from build123d import *

# Parameters (mm, degrees)
SKETCH1_R                = 2.159
BOSS_EXTRUDE2_DEPTH      = 2.54
BOSS_EXTRUDE5_DEPTH      = 25.4
BOSS_EXTRUDE5_DEPTH_BACK = 2.54
BOSS_EXTRUDE8_DEPTH      = 12.7
BOSS_EXTRUDE8_DEPTH_BACK = 2.54
SKETCH4_W                = 5.08
SKETCH4_H                = 2.54
BOSS_EXTRUDE9_DEPTH      = 5.08


with BuildPart() as part:
    # Sketch1 → Boss-Extrude2 (new body)
    with BuildSketch(Plane(origin=(0, 0, 0), x_dir=(1, 0, 0), z_dir=(0, 1, 0))):
        Polygon((0, -5.08), (5.08, -5.08), (10.489221848, 5.08), (43.764184298, 5.08), (51.562, -5.08), (61.722, -5.08), (61.722, 5.08), (56.642, 5.08), (51.562, 5.08), (46.152778152, 10.489221848), (10.489221848, 10.489221848), (5.08, 5.08), (-5.08, 5.08), (-5.08, -5.08), align=None)
        with Locations(Location((0, 0, 0), (0, 0, 270))):
            Circle(SKETCH1_R, mode=Mode.SUBTRACT)
        with Locations(Location((56.642, 0, 0), (0, 0, 270))):
            Circle(SKETCH1_R, mode=Mode.SUBTRACT)
    extrude(amount=BOSS_EXTRUDE2_DEPTH)

    # Sketch3 → Boss-Extrude5 (add, two sides: drawn at the far end of the back side and taken through both)
    with BuildSketch(Plane(origin=(0, 2.54, 0), x_dir=(1, 0, 0), z_dir=(0, 1, 0)).offset(-BOSS_EXTRUDE5_DEPTH_BACK)):
        Polygon((5.08, 12.7), (5.08, 5.08), (-5.08, 5.08), (-5.08, 12.7), (0, 12.7), align=None)
    extrude(amount=BOSS_EXTRUDE5_DEPTH + BOSS_EXTRUDE5_DEPTH_BACK)

    # Sketch4 → Boss-Extrude8 (add, two sides: drawn at the far end of the back side and taken through both)
    with BuildSketch(Plane(origin=(0, 2.54, 0), x_dir=(1, 0, 0), z_dir=(0, 1, 0)).offset(-BOSS_EXTRUDE8_DEPTH_BACK)):
        with Locations((29.878652905, 11.759221848)):
            Rectangle(SKETCH4_W, SKETCH4_H)
    extrude(amount=BOSS_EXTRUDE8_DEPTH + BOSS_EXTRUDE8_DEPTH_BACK)

    # Sketch7 → Boss-Extrude9 (add)
    with BuildSketch(Plane(origin=(32.418652905, 0, 0), x_dir=(0, 0, -1), z_dir=(1, 0, 0))):
        Polygon((10.489221848, 15.24), (5.391589044, 15.24), (5.391589044, 12.7), (5.391589044, 11.903510412), (7.271896049, 11.903510412), (8.703373283, 11.903510412), (8.703373283, 13.570272135), (7.703807283, 13.570272135), (7.703807283, 12.7), (7.271896049, 12.7), (6.661589044, 12.7), (5.865099456, 13.97), (6.661589044, 13.97), (10.489221848, 13.97), align=None)
    extrude(amount=-BOSS_EXTRUDE9_DEPTH)


solid = part.part
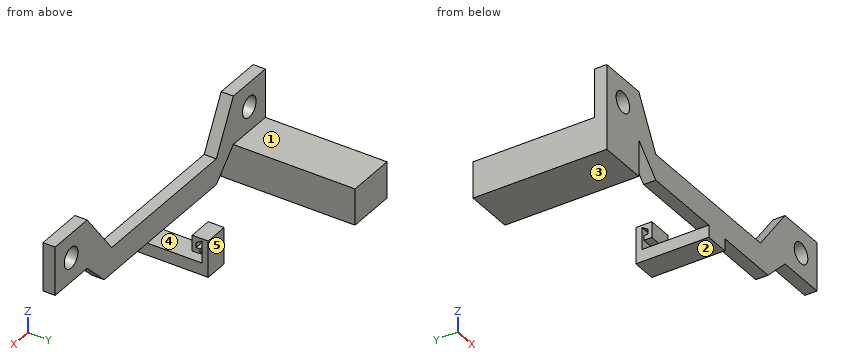
The model under review builds one solid part; all positions refer to its coordinate system, in mm. Face numbers are marked on the shaded views. A direction names the side the tool comes from. Coordinates: 2 decimals unless noted, no trailing zeros. Write each loop counter-clockwise with the first axis right and the second up, starting at its lowest first coordinate (ties: lowest second). Pieces come first, ordered by that corner, then holes. Notation, with made-up numbers: (40, -24.5) -> (97, -24.5) arc R4 ccw to (97, -17.5) -> close; hole circle Ø9 at (41, -24). An arc over 180 degrees is marked (long way). Answer in a Markdown table with one row per item.
1. For the marked faces 1 and 2, list the 3-axis set-ups (+Z, -Z, +X, -X, +Y, -Y) from which the entire face can be reached by the end or side of a thin tool; tool diameter is ignored.
Answers below:
| item | result |
|---|---|
| face 1 | +Z, +X, -X, +Y |
| face 2 | -Z, +X, -X, +Y, -Y |
2. Clearance check with flat-ended pins moving along their axes: pin 1 Ø2 at (x, y) = (56, 1) entering from -Z; pin 2 Ø6 at (y, z) = (8, -11) entering from +X; pin 3 Ø1 at (x, y) = (28.5, 13) entering from +Z. State where each tip first meets the part, or that it passes through.
Answers below:
| item | result |
|---|---|
| pin 1 | stops at z = -5.08 |
| pin 2 | stops at x = 32.42 |
| pin 3 | stops at z = -5.39 |
3. We need section D-D, the plane z = -9.5. State the section outline as (x, y) points.
Answers below:
| item | result |
|---|---|
| outline | (-5.08, 0) -> (5.08, 0) -> (5.08, 27.94) -> (-5.08, 27.94) -> close; (9.5, 0) -> (47.14, 0) -> (47.14, 2.54) -> (9.5, 2.54) -> close; (27.34, 13.97) -> (32.42, 13.97) -> (32.42, 15.24) -> (27.34, 15.24) -> close |
4. Draft analysis for pull direction Y (two halves, no side actions). For the marked faces 3, 4 and 5, state which applies: +Y half, -Y half, draft (parallel to the pull), parting line (faces both ways), or undercut.
Answers below:
| item | result |
|---|---|
| face 3 | draft |
| face 4 | undercut |
| face 5 | +Y half |
5. We need section B-B, the plane y = 9. State the section outline as (x, z) points.
Answers below:
| item | result |
|---|---|
| outline | (-5.08, -12.7) -> (5.08, -12.7) -> (5.08, -5.08) -> (-5.08, -5.08) -> close; (27.34, -13.03) -> (32.42, -13.03) -> (32.42, -10.49) -> (27.34, -10.49) -> close |
6. We need section A-A, the plane x = 0. State the section outline as (y, z) points, and give its area (3 significant figures).
Answers below:
| item | result |
|---|---|
| outline | (0, -12.7) -> (27.94, -12.7) -> (27.94, -5.08) -> (2.54, -5.08) -> (2.54, -2.16) -> (0, -2.16) -> close; (0, 2.16) -> (2.54, 2.16) -> (2.54, 5.08) -> (0, 5.08) -> close |
| area | 228 mm^2 |
7. We need section C-C, the plane z = -4.25. State the section outline as (x, y) points, and give its area (3 significant figures).
Answers below:
| item | result |
|---|---|
| outline | (-5.08, 0) -> (10.05, 0) -> (10.05, 2.54) -> (-5.08, 2.54) -> close; (44.4, 0) -> (61.72, 0) -> (61.72, 2.54) -> (44.4, 2.54) -> close |
| area | 82.4 mm^2 |
8. Wall thickness on probe 1 along X at (y, z) = (0.9, 0); probe 2 along Z at (x, y) = (3, 10); probe 3 along Y at (x, z) = (17.5, -7.5): over which ranges is each line inside the solid? List them lowest first. Write a range as [from, to].
Answers below:
| item | result |
|---|---|
| probe 1 | x = [-5.08, -2.16], [2.16, 7.78], [47.66, 54.48], [58.8, 61.72] |
| probe 2 | z = [-12.7, -5.08] |
| probe 3 | y = [0, 2.54] |
